```python
from build123d import *

# Parameters (mm, degrees)
FILLET1_R          = 3
FILLET2_R          = 0.75
SKETCH3_R          = 6.38
CUT_EXTRUDE1_DEPTH = 0.85


with BuildPart() as part:
    # Sketch2 → Revolve1 (revolve)
    with BuildSketch(Plane.XY):
        with BuildLine():
            Line((0, 263.525), (9.34, 263.525))
            Line((9.34, 263.525), (9.34, 243.380049267))
            Line((9.34, 243.380049267), (9.000677154, 242.525))
            Line((9.000677154, 242.525), (9.34, 241.669950733))
            Line((9.34, 241.669950733), (9.34, 3.410583034))
            ThreePointArc((9.34, 3.410583034), (9.391810091, 2.300465987), (9.546789941, 1.2))
            Line((9.546789941, 1.2), (9.000677154, 1.2))
            Line((9.000677154, 1.2), (9.000677154, 0))
            Line((9.000677154, 0), (0, 0))
            Line((0, 0), (0, 263.525))
        make_face()
    revolve(axis=Axis((0, 0, 0), (0, 1, 0)))

    # Fillet1
    fillet1_edges = [part.edges().sort_by_distance(p)[0] for p in [
        (-9.34, 263.525, 0),
    ]]
    fillet(fillet1_edges, radius=FILLET1_R)

    # Fillet2
    fillet2_edges = [part.edges().sort_by_distance(p)[0] for p in [
        (-9.000677154, 0, 0),
        (-9.34, 243.380049267, 0),
        (-9.000677154, 242.525, 0),
        (-9.34, 241.669950733, 0),
    ]]
    fillet(fillet2_edges, radius=FILLET2_R)

    # Sketch3 → Cut-Extrude1 (cut)
    with BuildSketch(Plane(origin=(0, 263.525, 0), x_dir=(1, 0, 0), z_dir=(0, 1, 0))):
        Circle(SKETCH3_R)
    extrude(amount=-CUT_EXTRUDE1_DEPTH, mode=Mode.SUBTRACT)


solid = part.part
```
Design review of the part built by this model. Coordinates are the model's own, in mm. A direction names the side the tool comes from. Give positions to 0.01 mm unless a question says otherwise; leave off trailing zeros. Write each loop counter-clockwise with the first axis right and the second up, starting at its lowest first coordinate (ties: lowest second). Pieces come first, ordered by that corner, then holes.
(1) Mouldability with a two-part tool opening along Z and no side actions: class faces 4 (the face through (-6, 1.2, -7)), 5 (the face through (4.31, 251.905, 8.286)), 6 (the face through (0, 262.675, 0)) as +Z half, -Z half, draft (parallel to the pull), parting line (faces both ways), or undercut.
Checked values:
face 4: draft
face 5: parting line
face 6: undercut
(2) Add section A-A (y = 131.5). Give the boundary of the cut face in (x, z), and give its area (3 significant figures).
Checked values:
outline: circle Ø18.68 at (0, 0)
area: 274 mm2
(3) Clearance check with flat-ended pins moving along their axes: pin 1 Ø5 at (x, y) = (-0.5, 85) entering from +Z; pin 2 Ø5.5 at (x, z) = (0.5, -1.5) entering from -Y; pin 3 Ø2 at (y, z) = (193, -4.5) entering from -X; pin 4 Ø1.5 at (x, y) = (-6.5, 237) entering from +Z. State where each tip first meets the part, or that it passes through.
Checked values:
pin 1: stops at z = 9.34
pin 2: stops at y = 0
pin 3: stops at x = -8.66
pin 4: stops at z = 7.36
(4) Wall thickness on line 1 along Z through (x, y) = (-0.25, 119.5); line 2 along Y through (x, z) = (4.75, 5); line 3 along Z through (x, y) = (0, 263.2): over which ranges is each line inside the solid? List them lowest first.
Checked values:
line 1: z = -9.34 to 9.34
line 2: y = 0 to 263.47
line 3: z = -7.7 to -6.38, 6.38 to 7.7
(5) Tool access review of faces 1 (the face through (0, 0, 0)), 2 (the face through (8.628, 120.802, 3.577)), 3 (the face through (4.84, 0.97, -7.59)): name each direction out of +Z, -Z, +X, -X, +Y, -Y from which nothing blocks a thin tool from reaching the whole face with its end or side.
Checked values:
face 1: +Z, -Z, +X, -X, -Y
face 2: +Y
face 3: -Y
